Source: CAD feature listing. Evaluate the final solid. Frame: model axes, mm. A direction names the side the tool comes from. Give positions to 0.01 mm unless a question says otherwise; leave off trailing zeros. Loops run counter-clockwise (first coordinate to the right, second up) from the corner with the lowest first, then second, coordinate; pieces in that order, holes last. Notation, with made-up numbers: (10, 78) -> (51, 78) arc R34 cw to (51, 116) -> close; hole circle Ø11 at (18, 2). An arc over 180 degrees is marked (long way). Return JSON: item names as keys, results as strings. Group by question number.
(1) Draft query along X for faces 1 (the face through (3.824, 0.496, 0.986)), 2 (the face through (12.844, -0.049, 1.261)), 3 (the face through (-4.75, 0.04, 0.99)), 4 (the face through (-2, 1, 2)). Return one class per face: released by +X, released by -X, zero draft, split by the parting line, or undercut.
(2) Cut plane C-C on x = 2.25. Return loops of the section in (y, z).
(3) Cut plane D-D on y = -3. Return loops of the section in (x, z), then the cut area to 3 significant figures.
(4) Ray query, line 1 (X direction, y = 0.5, z = 1.1); line 2 (X direction, y = 0.25, z = 1.4); line 3 (Y direction, x = -1.25, z = 1). Return the intervals inside material, ascending. Write a range as from..to.
(5) Cut plane A-A on x = -1.25. Return loops of the section in (y, z).
(6) Cut plane B-B on y = 0. Return loops of the section in (x, z).
(7) Access query for faces 5 (the face through (10.25, 0, 2.5)), 6 (the face through (-13.75, 0, 1)), 7 (the face through (11.25, 0, 2.5)). Directions: +Z, -Z, +X, -X, +Y, -Y. A direction counts if a zero-diameter tool reaches every point of the face in a straight line with its end or side. Return the directions, or none.
(8) Pin query (flat end, axial travel): pin 1 (0.5 mm diameter, centred on y = 0, z = 2.5, fed in from -X); pin 2 (4 mm diameter, centred on x = 2.25, y = 0, fed in from +Z); pin 3 (1.1 mm diameter, centred on y = 1.5, z = 2.5, fed in from +X); pin 4 (1.2 mm diameter, centred on x = -1.25, y = 0, fed in from -Z). Return the tip coordinate at first contact, or that it passes through.
```python
from build123d import *

# Parameters (mm, degrees)
ESBO_O1_W                = 27.5
ESBO_O1_H                = 7
ESBO_O1_R                = 1.65
ESBO_O1_R_2              = 1
RESSALTO_EXTRUS_O1_DEPTH = 2
CHANFRO1_SIZE            = 1.5
CHANFRO1_SIZE2           = 1.787630389
ESBO_O2_W                = 1
ESBO_O2_H                = 7
RESSALTO_EXTRUS_O2_DEPTH = 1


with BuildPart() as part:
    # Esboço1 → Ressalto-extrusão1 (new body)
    with BuildSketch(Plane.XY):
        Rectangle(ESBO_O1_W, ESBO_O1_H)
        with Locations((2.25, 0)):
            Circle(ESBO_O1_R, mode=Mode.SUBTRACT)
        with Locations((-1.25, 0)):
            Circle(ESBO_O1_R_2, mode=Mode.SUBTRACT)
        with Locations((-3.75, 0)):
            Circle(ESBO_O1_R_2, mode=Mode.SUBTRACT)
    extrude(amount=RESSALTO_EXTRUS_O1_DEPTH)

    # Chanfro1
    chanfro1_edges = [part.edges().sort_by_distance(p)[0] for p in [
        (13.75, 0, 2),
    ]]
    chanfro1_side = [part.faces().sort_by_distance(p)[0] for p in [
        (13.75, 0, 1),
    ]]
    chamfer(chanfro1_edges, length=CHANFRO1_SIZE, length2=CHANFRO1_SIZE2, reference=chanfro1_side[0])

    # Esboço2 → Ressalto-extrusão2 (add)
    with BuildSketch(Plane.XY.offset(2)):
        with Locations((10.75, 0)):
            Rectangle(ESBO_O2_W, ESBO_O2_H)
    extrude(amount=RESSALTO_EXTRUS_O2_DEPTH)


solid = part.part
```
Answers:
{
 "1": {"face 1": "undercut", "face 2": "released by +X", "face 3": "undercut", "face 4": "zero draft"},
 "2": {"outline": "(-3.5, 0) -> (-1.65, 0) -> (-1.65, 2) -> (-3.5, 2) -> close; (1.65, 0) -> (3.5, 0) -> (3.5, 2) -> (1.65, 2) -> close"},
 "3": {"outline": "(-13.75, 0) -> (13.75, 0) -> (13.75, 0.5) -> (11.96, 2) -> (11.25, 2) -> (11.25, 3) -> (10.25, 3) -> (10.25, 2) -> (-13.75, 2) -> close", "area": "54.7 mm²"},
 "4": {"line 1": "-13.75..-4.62, -2.88..-2.12, -0.38..0.68, 3.82..13.03", "line 2": "-13.75..-4.72, -2.78..-2.22, -0.28..0.62, 3.88..12.68", "line 3": "-3.5..-1, 1..3.5"},
 "5": {"outline": "(-3.5, 0) -> (-1, 0) -> (-1, 2) -> (-3.5, 2) -> close; (1, 0) -> (3.5, 0) -> (3.5, 2) -> (1, 2) -> close"},
 "6": {"outline": "(-13.75, 0) -> (-4.75, 0) -> (-4.75, 2) -> (-13.75, 2) -> close; (-2.75, 0) -> (-2.25, 0) -> (-2.25, 2) -> (-2.75, 2) -> close; (-0.25, 0) -> (0.6, 0) -> (0.6, 2) -> (-0.25, 2) -> close; (3.9, 0) -> (13.75, 0) -> (13.75, 0.5) -> (11.96, 2) -> (11.25, 2) -> (11.25, 3) -> (10.25, 3) -> (10.25, 2) -> (3.9, 2) -> close"},
 "7": {"face 5": "+Z, -X, +Y, -Y", "face 6": "+Z, -Z, -X, +Y, -Y", "face 7": "+Z, +X, +Y, -Y"},
 "8": {"pin 1": "x = 10.25", "pin 2": "z = 2", "pin 3": "x = 12.02", "pin 4": "through"}
}
